from build123d import *

# Parameters (mm, degrees)
SKETCH1_W               = 59
SKETCH1_H               = 102.5
BOSS_EXTRUDE1_DEPTH     = 2
SKETCH2_W               = 63
SKETCH2_H               = 106.5
SKETCH2_W_2             = 59
SKETCH2_H_2             = 102.5
BOSS_EXTRUDE2_DEPTH     = 12.6
SKETCH4_W               = 59
SKETCH4_H               = 3
SKETCH4_W_2             = 3
SKETCH4_W_3             = 15
SKETCH4_H_2             = 23
SKETCH4_W_4             = 6
SKETCH4_H_3             = 17
SKETCH4_H_4             = 10
SKETCH4_W_5             = 5
BOSS_EXTRUDE3_DEPTH     = 4
CUT_EXTRUDE1_REACH      = 125.378
SKETCH5_W               = 20
SKETCH5_H               = 6
SKETCH5_W_2             = 10.8
SKETCH5_H_2             = 4
CHAMFER1_SIZE           = 0.5
CHAMFER2_SIZE           = 1
SKETCH6_W               = 2
SKETCH6_H               = 1.3
CUT_EXTRUDE2_DEPTH      = 20
CUT_EXTRUDE3_DEPTH      = 122.655291706
CUT_EXTRUDE3_DEPTH_BACK = 122.655291706
SKETCH7_W               = 60.5
SKETCH7_H               = 3
CHAMFER3_SIZE           = 3


with BuildPart() as part:
    # Sketch1 → Boss-Extrude1 (new body)
    with BuildSketch(Plane(origin=(0, 0, 0), x_dir=(1, 0, 0), z_dir=(0, 1, 0))):
        with Locations((29.5, -51.25)):
            Rectangle(SKETCH1_W, SKETCH1_H)
    extrude(amount=BOSS_EXTRUDE1_DEPTH)

    # Sketch2 → Boss-Extrude2 (add)
    with BuildSketch(Plane(origin=(0, 0, 0), x_dir=(1, 0, 0), z_dir=(0, 1, 0))):
        with Locations((29.5, -51.25)):
            Rectangle(SKETCH2_W, SKETCH2_H)
        with Locations((29.5, -51.25)):
            Rectangle(SKETCH2_W_2, SKETCH2_H_2, mode=Mode.SUBTRACT)
    extrude(amount=BOSS_EXTRUDE2_DEPTH)

    # Sketch4 → Boss-Extrude3 (add)
    with BuildSketch(Plane(origin=(0, 2, 0), x_dir=(1, 0, 0), z_dir=(0, 1, 0))):
        with Locations((29.5, -83)):
            Rectangle(SKETCH4_W, SKETCH4_H)
        with Locations((29.5, -64)):
            Rectangle(SKETCH4_W, SKETCH4_H)
        with Locations((16.5, -101)):
            Rectangle(SKETCH4_W_2, SKETCH4_H)
        with Locations((35.5, -101)):
            Rectangle(SKETCH4_W_2, SKETCH4_H)
        with Locations((54.5, -101)):
            Rectangle(SKETCH4_W_2, SKETCH4_H)
        with Locations((7.5, -35)):
            Rectangle(SKETCH4_W_3, SKETCH4_H_2)
        with Locations((56, -38)):
            Rectangle(SKETCH4_W_4, SKETCH4_H_3)
        with Locations((57.5, -5)):
            Rectangle(SKETCH4_W_2, SKETCH4_H_4)
        with Locations((25.5, -17)):
            Rectangle(SKETCH4_W_5, SKETCH4_H_4)
    extrude(amount=BOSS_EXTRUDE3_DEPTH)

    # Sketch5 → Cut-Extrude1 (cut, up to next)
    with BuildSketch(Plane(origin=(0, 0, -2), x_dir=(-1, 0, 0), z_dir=(0, 0, -1)), mode=Mode.PRIVATE) as cut_extrude1_sk1:
        with Locations((-11.5, 7.5)):
            Rectangle(SKETCH5_W, SKETCH5_H)
    cut_extrude1_tool1 = extrude(cut_extrude1_sk1.sketch, amount=-CUT_EXTRUDE1_REACH, mode=Mode.PRIVATE) & part.part
    # Sketch5 → Cut-Extrude1 (cut, up to next)
    with BuildSketch(Plane(origin=(0, 0, -2), x_dir=(-1, 0, 0), z_dir=(0, 0, -1)), mode=Mode.PRIVATE) as cut_extrude1_sk2:
        with Locations((-47.9, 4.5)):
            Rectangle(SKETCH5_W_2, SKETCH5_H_2)
    cut_extrude1_tool2 = extrude(cut_extrude1_sk2.sketch, amount=-CUT_EXTRUDE1_REACH, mode=Mode.PRIVATE) & part.part
    add(cut_extrude1_tool1.solids().sort_by_distance((11.5, 7.5, -2))[0], mode=Mode.SUBTRACT)
    add(cut_extrude1_tool2.solids().sort_by_distance((47.9, 4.5, -2))[0], mode=Mode.SUBTRACT)

    # Chamfer1
    chamfer1_edges = [part.edges().sort_by_distance(p)[0] for p in [
        (18, 2, 101),
        (15, 2, 101),
        (16.5, 2, 99.5),
        (37, 2, 101),
        (34, 2, 101),
        (35.5, 2, 99.5),
        (56, 2, 101),
        (53, 2, 101),
        (54.5, 2, 99.5),
        (29.5, 2, 84.5),
        (29.5, 2, 81.5),
        (28, 2, 17),
        (25.5, 2, 22),
        (23, 2, 17),
        (25.5, 2, 12),
        (56, 2, 5),
        (57.5, 2, 10),
        (56, 2, 46.5),
        (53, 2, 38),
        (56, 2, 29.5),
        (7.5, 2, 23.5),
        (15, 2, 35),
        (7.5, 2, 46.5),
        (29.5, 2, 65.5),
        (29.5, 2, 62.5),
    ]]
    chamfer(chamfer1_edges, length=CHAMFER1_SIZE)

    # Chamfer2
    chamfer2_edges = [part.edges().sort_by_distance(p)[0] for p in [
        (-2, 0, 51.25),
        (-2, 6.3, 104.5),
        (29.5, 0, -2),
        (-2, 6.3, -2),
        (61, 0, 51.25),
        (61, 6.3, -2),
        (29.5, 0, 104.5),
        (61, 6.3, 104.5),
        (53.3, 4.5, -2),
        (47.9, 2.5, -2),
        (42.5, 4.5, -2),
        (47.9, 6.5, -2),
    ]]
    chamfer(chamfer2_edges, length=CHAMFER2_SIZE)

    # Sketch6 → Cut-Extrude2 (cut)
    with BuildSketch(Plane.XY):
        with Locations((-1, 10.25)):
            Rectangle(SKETCH6_W, SKETCH6_H)
        with Locations((60, 10.25)):
            Rectangle(SKETCH6_W, SKETCH6_H)
    extrude(amount=CUT_EXTRUDE2_DEPTH, mode=Mode.SUBTRACT)

    # Sketch7 → Cut-Extrude3 (cut, two sides: drawn at the far end of the back side and taken through both)
    with BuildSketch(Plane(origin=(0, 0, 0), x_dir=(0, 0, -1), z_dir=(1, 0, 0)).offset(-CUT_EXTRUDE3_DEPTH_BACK)):
        with Locations((-74.25, 11.1)):
            Rectangle(SKETCH7_W, SKETCH7_H)
    extrude(amount=CUT_EXTRUDE3_DEPTH + CUT_EXTRUDE3_DEPTH_BACK, mode=Mode.SUBTRACT)

    # Chamfer3
    chamfer3_edges = [part.edges().sort_by_distance(p)[0] for p in [
        (-1, 12.6, 44),
        (60, 12.6, 44),
    ]]
    chamfer(chamfer3_edges, length=CHAMFER3_SIZE - 0.0001)  # a hair under: the kernel refuses the full size


solid = part.part
Verification items for the finished model (mm, model axes). A direction names the side the tool comes from. Coordinates: 2 decimals unless noted, no trailing zeros. Order: outer loops, then holes, each group sorted by start corner. A loop starts at its lowest first (then second) coordinate and runs counter-clockwise, first axis right, second up. Notation, with made-up numbers: (14.25, 79.5) -> (61.25, 79.5) arc R35 ccw to (61.25, 115.5) -> close; hole circle Ø3 at (56.5, 80.25). An arc over 180 degrees is marked (long way). Put each result on its own line as item: value. Start each with the question number.
1. Mould release check, pull along Z, two halves, no side actions. Record for faces 1 (the flat face through (29, 0, 51)), 2 (the flat face through (29, 7, -2)), 3 (the flat face through (15, 4, 35)): released by +Z, released by -Z, zero draft, split by the parting line, or undercut.
2. Go/stop test with flat-tipped pins: pin 1 Ø0.9 at (x, z) = (16.5, 101.5) entering from +Y; pin 2 Ø1.5 at (x, z) = (29, 46) entering from +Y. Record where each tip stops, or that it passes through.
3. Access from +Z, -Z, +X, -X, +Y, -Y to the whole of each face (thin tool, end or side, straight path). Record for faces 4 (the flat face through (35, 4, 99.5)), 5 (the flat face through (-1, 10.9, 10)), 6 (the flat face through (29, 9.6, 104)).
4. Cross-section at A-A, the plane z = 17. Record the boundary of the cut face in (x, y), then the cut area to 3 significant figures.
5. Material ranges on L1, parallel to X at y = 4.25, z = 14.5; L2, parallel to Z at x = 55, y = 5; L3, parallel to X at y = 9.5, z = 43, recorded low to high. Write a range as [from, to].
6. Cross-section at C-C, the plane x = 30.5. Record the boundary of the cut face in (y, z), then the cut area to 3 significant figures.
7. Cross-section at D-D, the plane z = 90. Record the boundary of the cut face in (x, y), then the cut area to 3 significant figures.
Computed:
1. face 1: zero draft
1. face 2: released by -Z
1. face 3: undercut
2. pin 1: y = 6
2. pin 2: y = 2
3. face 4: +Y
3. face 5: +X, -X
3. face 6: +Z, +X, -X, +Y
4. outline: (-2, 1) -> (-1, 0) -> (60, 0) -> (61, 1) -> (61, 9.6) -> (59, 9.6) -> (59, 2) -> (28.5, 2) -> (28, 2.5) -> (28, 6) -> (23, 6) -> (23, 2.5) -> (22.5, 2) -> (0, 2) -> (0, 9.6) -> (-2, 9.6) -> close; (-2, 10.9) -> (0, 10.9) -> (0, 12.6) -> (-2, 12.6) -> close; (59, 10.9) -> (61, 10.9) -> (61, 12.6) -> (59, 12.6) -> close
4. area: 182 mm2
5. L1: [-2, 0], [23, 28], [59, 61]
5. L2: [-2, 0], [29.5, 46.5], [62.5, 65.5], [81.5, 84.5], [99.5, 104.5]
5. L3: [-2, 0], [59, 61]
6. outline: (0, -1) -> (1, -2) -> (12.6, -2) -> (12.6, 0) -> (2, 0) -> (2, 62) -> (2.5, 62.5) -> (6, 62.5) -> (6, 65.5) -> (2.5, 65.5) -> (2, 66) -> (2, 81) -> (2.5, 81.5) -> (6, 81.5) -> (6, 84.5) -> (2.5, 84.5) -> (2, 85) -> (2, 102.5) -> (9.6, 102.5) -> (9.6, 104.5) -> (1, 104.5) -> (0, 103.5) -> close
6. area: 273 mm2
7. outline: (-2, 1) -> (-1, 0) -> (60, 0) -> (61, 1) -> (61, 9.6) -> (59, 9.6) -> (59, 2) -> (0, 2) -> (0, 9.6) -> (-2, 9.6) -> close
7. area: 155 mm2
